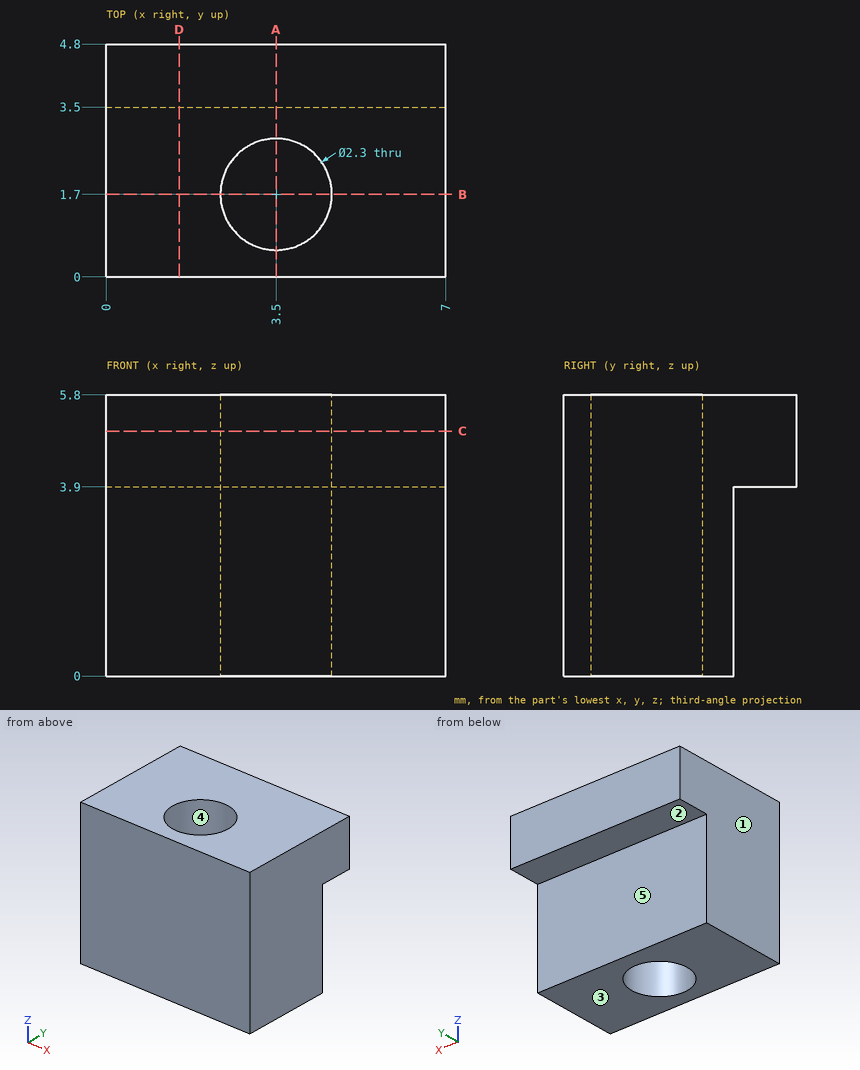
Drawing for the job (mm, zero at the part's lowest x, y, z). A direction names the side the tool comes from. Coordinates: 2 decimals unless noted, no trailing zeros. Order: outer loops, then holes, each group sorted by start corner. A loop starts at its lowest first (then second) coordinate and runs counter-clockwise, first axis right, second up.
Item 1: Band-saw the part on B-B on y = 1.7. List the corners of the cut face in (x, z), plus the area to 3 significant figures.
Check sheet entries:
outline: (0, 0) - (2.35, 0) - (2.35, 5.8) - (0, 5.8) - close; (4.65, 0) - (7, 0) - (7, 5.8) - (4.65, 5.8) - close
area: 27.3 mm2
Item 2: Band-saw the part on C-C on z = 5.05. List the corners of the cut face in (x, y).
Check sheet entries:
outline: (0, 0) - (7, 0) - (7, 4.8) - (0, 4.8) - close; hole circle Ø2.3 at (3.5, 1.7)
Item 3: Two-plate mould, pull along Y, no slides. Class the marked faces 3, 4 and 5: +Y half, -Y half, draft (parallel to the pull), parting line (faces both ways), or undercut.
Check sheet entries:
face 3: draft
face 4: undercut
face 5: +Y half
Item 4: Pin check, flat tip, straight feed: pin 1 Ø2 at (x, y) = (3.5, 1.7) entering from +Z. Stop position of the tip, or through.
Check sheet entries:
pin 1: passes through
Item 5: 3-axis set-ups, long thin cutter, end or side, ignore diameter. For the marked faces 1 and 2: which of +Z, -Z, +X, -X, +Y, -Y reach the whole face in a straight line?
Check sheet entries:
face 1: +Z, -Z, -X, +Y, -Y
face 2: -Z, +X, -X, +Y
Item 6: Band-saw the part on D-D on x = 1.5. List the corners of the cut face in (y, z), plus the area to 3 significant figures.
Check sheet entries:
outline: (0, 0) - (3.5, 0) - (3.5, 3.9) - (4.8, 3.9) - (4.8, 5.8) - (0, 5.8) - close
area: 22.8 mm2
Item 7: Drill centre lines: L1, parallel to Y at x = 3.5, z = 5.5; L2, parallel to Y at x = 3.5, z = 3.75; L3, parallel to X at y = 1.65, z = 1.4. Where is each one in solid material? Low to high.
Check sheet entries:
L1: y = 0 to 0.55, 2.85 to 4.8
L2: y = 0 to 0.55, 2.85 to 3.5
L3: x = 0 to 2.35, 4.65 to 7
Item 8: Band-saw the part on A-A on x = 3.5. List the corners of the cut face in (y, z).
Check sheet entries:
outline: (0, 0) - (0.55, 0) - (0.55, 5.8) - (0, 5.8) - close; (2.85, 0) - (3.5, 0) - (3.5, 3.9) - (4.8, 3.9) - (4.8, 5.8) - (2.85, 5.8) - close
